from build123d import *


with BuildPart() as part:
    # Esboço2 → Revolução1 (revolve)
    with BuildSketch(Plane.XY):
        with BuildLine():
            Line((1.25, 6.25), (13.75, 6.25))
            Line((13.75, 6.25), (13.75, 7.5))
            Line((13.75, 7.5), (12.5, 10))
            Line((12.5, 10), (12.5, 12.5))
            Line((12.5, 12.5), (15, 15))
            Line((15, 15), (15, 22.5))
            Line((15, 22.5), (12.5, 22.5))
            Line((12.5, 22.5), (12.5, 19.5))
            ThreePointArc((12.5, 19.5), (11.914213562, 18.085786438), (10.5, 17.5))
            Line((10.5, 17.5), (4.5, 17.5))
            ThreePointArc((4.5, 17.5), (3.085786438, 18.085786438), (2.5, 19.5))
            Line((2.5, 19.5), (2.5, 22.5))
            Line((2.5, 22.5), (0, 22.5))
            Line((0, 22.5), (0, 15))
            Line((0, 15), (2.5, 12.5))
            Line((2.5, 12.5), (2.5, 10))
            Line((2.5, 10), (1.25, 7.5))
            Line((1.25, 7.5), (1.25, 6.25))
        make_face()
    revolve(axis=Axis((0, 0, 0), (1, 0, 0)))


solid = part.part
Source: CAD feature listing. Evaluate the final solid. Frame: model axes, mm. A direction names the side the tool comes from. Give positions to 0.01 mm unless a question says otherwise; leave off trailing zeros. Write each loop counter-clockwise with the first axis right and the second up, starting at its lowest first coordinate (ties: lowest second). Pieces come first, ordered by that corner, then holes. Notation, with made-up numbers: (-27, 11.5) - (-10, 11.5) arc R18 cw to (-10, 30.5) - close; hole circle Ø10 at (81, 29.5). An arc over 180 degrees is marked (long way). Write item = value, one per line. Start each with the question number.
Q1. Reachability of faces 1 (the flat face through (12.5, -17, 10)), 2 (the flat face through (1.25, -3, 6)), 3 (the flat face through (13.75, 3, 6)) from +Z, -Z, +X, -X, +Y, -Y: full face, straight path, thin tool, end or side. Return the list, or none.
Q2. Draft query along Z for faces 4 (the flat face through (2.5, -0.1, 10.2)), 5 (the flat face through (0, 15, -5)), 6 (the flat face through (12.5, 0.1, 10.2)), 7 (the cylindrical face through (7.458, -13.887, -10.648)). Return one class per face: +Z half, -Z half, draft (parallel to the pull), parting line (faces both ways), or undercut.
Q3. Cut plane B-B, the plane x = 3.5. Return loops of the section in (y, z), then the cut area to 3 significant figures.
Q4. Material intervals for probe 1 along X at (y, z) = (13, 15); probe 2 along Y at (x, z) = (13.5, -1); probe 3 along Z at (x, y) = (8.75, 0), sorted ascending.
Q5. Cut plane A-A, the plane x = 6. Return loops of the section in (y, z).
Q6. Pin query (flat end, axial travel): pin 1 Ø8 at (x, z) = (11, 5.5) entering from -Y; pin 2 Ø5 at (x, z) = (8, -12) entering from +Y; pin 3 Ø3 at (y, z) = (-7.5, -2) entering from +X; pin 4 Ø20 at (y, z) = (5.5, -4.5) entering from +X. Return the tip coordinate at first contact, or that it passes through.
Computed values:
q1.face_1 = none
q1.face_2 = -X
q1.face_3 = +X
q2.face_4 = undercut
q2.face_5 = draft
q2.face_6 = undercut
q2.face_7 = parting line
q3.outline = circle Ø35.54 at (0, 0); hole circle Ø12.5 at (0, 0)
q3.area = 869 mm²
q4.probe_1 = 0 to 2.5, 12.5 to 15
q4.probe_2 = -22.48 to -13.46, -7.94 to -6.17, 6.17 to 7.94, 13.46 to 22.48
q4.probe_3 = -17.5 to -6.25, 6.25 to 17.5
q5.outline = circle Ø35 at (0, 0); hole circle Ø12.5 at (0, 0)
q6.pin_1 = -22.43
q6.pin_2 = 14.7
q6.pin_3 = 13.75
q6.pin_4 = 15
